Could you check a few things on this model? Use its own coordinates, in mm. A direction names the side the tool comes from. Coordinates: 2 decimals unless noted, no trailing zeros. Loops run counter-clockwise (first coordinate to the right, second up) from the corner with the lowest first, then second, coordinate; pieces in that order, holes last. Notation, with made-up numbers: (20.25, 26.25) -> (56.25, 26.25) arc R17 ccw to (56.25, 32.25) -> close; hole circle Ø4 at (36, 84). An arc over 180 degrees is marked (long way). One line per question, with ' | ' between items.
```python
from build123d import *

# Parameters (mm, degrees)
SKETCH1_W           = 95.25
SKETCH1_H           = 95.25
SKETCH1_R           = 7.14375
BOSS_EXTRUDE1_DEPTH = 6.35
SKETCH3_R           = 19.05
SKETCH3_R_2         = 7.14375
BOSS_EXTRUDE2_DEPTH = 6.35
SKETCH2_R           = 14.2875
CUT_EXTRUDE1_DEPTH  = 7.9375
SKETCH4_R           = 8.73125
CUT_EXTRUDE2_DEPTH  = 3.175


with BuildPart() as part:
    # Sketch1 → Boss-Extrude1 (new body)
    with BuildSketch(Plane(origin=(0, 0, 0), x_dir=(1, 0, 0), z_dir=(0, 1, 0))):
        Rectangle(SKETCH1_W, SKETCH1_H)
        Circle(SKETCH1_R, mode=Mode.SUBTRACT)
    extrude(amount=BOSS_EXTRUDE1_DEPTH)

    # Sketch3 → Boss-Extrude2 (add)
    with BuildSketch(Plane(origin=(0, 6.35, 0), x_dir=(1, 0, 0), z_dir=(0, 1, 0))):
        Circle(SKETCH3_R)
        Circle(SKETCH3_R_2, mode=Mode.SUBTRACT)
    extrude(amount=BOSS_EXTRUDE2_DEPTH)

    # Sketch2 → Cut-Extrude1 (cut)
    with BuildSketch(Plane.XZ):
        Circle(SKETCH2_R)
    extrude(amount=-CUT_EXTRUDE1_DEPTH, mode=Mode.SUBTRACT)

    # Sketch4 → Cut-Extrude2 (cut)
    with BuildSketch(Plane(origin=(0, 12.7, 0), x_dir=(1, 0, 0), z_dir=(0, 1, 0))):
        Circle(SKETCH4_R)
    extrude(amount=-CUT_EXTRUDE2_DEPTH, mode=Mode.SUBTRACT)


solid = part.part
```
Q1. Imagine slicing it at D-D on x = -40. Write out the boundary of the cut face in (y, z) (3 decimals).
Values follow:
outline: (0, -47.625) -> (6.35, -47.625) -> (6.35, 47.625) -> (0, 47.625) -> close
Q2. For faces 4 (the face through (-7, 7.938, -3)), 5 (the face through (-15.12, 9.48, 11.59)), 6 (the face through (-1, 3, -47.625)), which set-ups out of +Z, -Z, +X, -X, +Y, -Y let a thin tool reach every point of the face, with its end or its side?
Values follow:
face 4: -Y | face 5: +Y | face 6: -Z, +X, -X, +Y, -Y
Q3. Imagine slicing it at C-C on y = 3.25. Write out the boundary of the cut face in (x, z) (1 decimal), plus the area to 3 significant figures.
Values follow:
outline: (-47.6, -47.6) -> (47.6, -47.6) -> (47.6, 47.6) -> (-47.6, 47.6) -> close; hole circle Ø28.6 at (0, 0) | area: 8,430 mm2
Q4. For pin 1 (8.5 mm diameter, centred on x = -5.5, z = -4, fed in from -Y); pin 2 (2 mm diameter, centred on x = 18, y = 9, fed in from +Z); pin 3 (3 mm diameter, centred on x = 24.5, z = 35.5, fed in from +Y); pin 4 (10 mm diameter, centred on x = 25, z = -26, fed in from -Y), each with a flat end and sliding along its axis, tell me the tip position at first contact or that it passes through.
Values follow:
pin 1: stops at y = 7.94 | pin 2: stops at z = 8.6 | pin 3: stops at y = 6.35 | pin 4: stops at y = 0
Q5. We'd pull the mould along Z, two halves only. Please class faces 1 (the face through (8, 12.7, 4)), 2 (the face through (-1, 3, 47.625)), 3 (the face through (-14.274, 3.913, 0.628)): released by +Z, released by -Z, zero draft, split by the parting line, or undercut.
Values follow:
face 1: zero draft | face 2: released by +Z | face 3: undercut
Q6. Please list where these lines run through material, in increasing order: L1, parallel to Z at x = 0, y = 9.15; L2, parallel to X at y = 10.9, z = 0. Write a range as [from, to].
Values follow:
L1: z = [-19.05, -7.14], [7.14, 19.05] | L2: x = [-19.05, -8.73], [8.73, 19.05]
